The listing builds one solid part. Answer for the finished solid, in the listing's coordinates (mm). Face numbers are marked on the shaded views. A direction names the side the tool comes from. Give positions to 0.01 mm unless a question says otherwise; leave off trailing zeros. Write each loop counter-clockwise with the first axis right and the second up, starting at its lowest first coordinate (ties: lowest second). Pieces come first, ordered by that corner, then holes. Notation, with made-up numbers: (-23.75, 48.25) -> (-8.75, 48.25) arc R16 ccw to (-8.75, 53.25) -> close; hole circle Ø3 at (76.25, 68). An arc over 180 degrees is marked (long way). Use CSV: the item, a comma, the result in double quotes. Start each with the question number.
Autodesk Inventor part; units mm, degrees
ref_plane "Work Plane1" through (10, 0, 10) normal (0.7071, 0, -0.7071) x (0, -1, 0)
ref_plane "Work Plane2" through (0, -10, 0) normal (0, 1, 0) x (1, 0, 0)
ref_plane "YZ Plane" through (0, 0, 0) normal (1, 0, 0) x (0, 1, 0)
sketch "Sketch1" plane through (0, 0, 0) normal (0, 1, 0) x (-1, 0, 0)
  line L0 (10, -10) -> (-10, -10)
  line L1 (-10, -10) -> (-10, 10)
  line L2 (-10, 10) -> (10, 10)
  line L3 (10, 10) -> (10, -10)
  dimension "d0" = 20
  dimension "d1" = 20
extrude "Main Body Extrusion" add sketch "Sketch1" against normal blind 10
ref_plane "Work Plane1" through (10, 0, 10) normal (0.7071, 0, -0.7071) x (0, -1, 0)
sketch "Sketch2" plane through (10, 0, 10) normal (0.7071, 0, -0.7071) x (0, -1, 0)
  line L0 (0, 0) -> (10, 0)
  line L1 (10, 14.1421) -> (10, 28.2843)
  line L2 (5, 0) -> (10, 28.2843)
  line L3 (5, 0) -> (10, 0)
  line L4 (10, 0) -> (10, 14.1421)
  line L5 (10, 14.1421) -> (10, 0)
  point P0 (0, 14.1421)
extrude "Slanted Cut" cut sketch "Sketch2" along normal through all both and the other way through all
sketch "Sketch3" plane through (0, 0, 0) normal (0, 1, 0) x (1, 0, 0)
  point P0 (0, 0)
  point P1 (0, 0)
hole "Screw Hole" at (0, 0, 0) direction (0, -1, 0) diameter 4.2 end through all
ref_plane "Work Plane2" through (0, -10, 0) normal (0, 1, 0) x (1, 0, 0)
sketch "Sketch4" plane through (0, -10, 0) normal (0, 1, 0) x (1, 0, 0)
  circle A0 centre (0, 0) radius 4
  dimension "d14" = 8
extrude "Counterbore for Screw Hole" cut sketch "Sketch4" along normal blind 7.5
sketch "Sketch5" plane through (0, 0, 0) normal (0, 1, 0) x (1, 0, 0)
  line L0 (-10, -10) -> (10, -10)
  line L1 (3, -10) -> (-3, -10)
  line L2 (-3, -10) -> (-3, 10)
  line L3 (-3, 10) -> (3, 10)
  line L4 (3, 10) -> (3, -10)
  circle A0 centre (0, 0) radius 2.1
  line L5 (3, 10) -> (-3, 10)
  line L6 (-3, 10) -> (-3, 6)
  line L7 (-3, 6) -> (3, 6)
  line L8 (3, 6) -> (3, 10)
  line L9 (3, -10) -> (-3, -10)
  line L10 (-3, -10) -> (-3, -6)
  line L11 (-3, -6) -> (3, -6)
  line L12 (3, -6) -> (3, -10)
extrude "Alignment Extrusion" add sketch "Sketch5" along normal blind 3 contours L2 L11 L4 L0 | L2 L3 L4 L7
properties part number "corner_3DPrint"
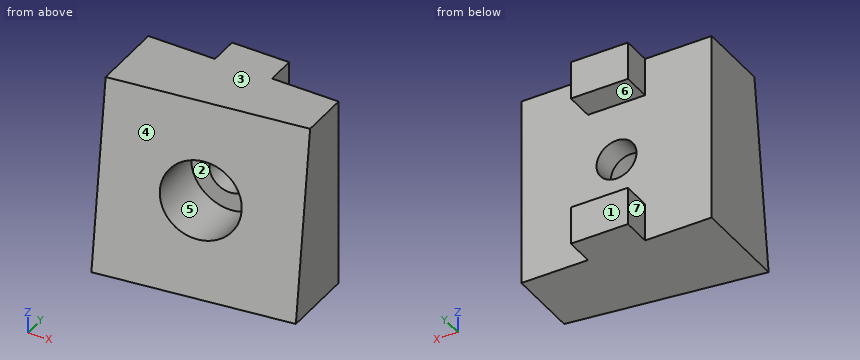
Q1. The mould has two halves that part along Z. Classify the marked faces 1, 2 and 3: +Z half, -Z half, draft (parallel to the pull), parting line (faces both ways), or undercut.
Q2. Section C-C on y = 0.75 is taken. Give the vertices of the cut face in (x, z), then the cut area to 3 significant figures.
Q3. Section B-B on z = 0 is taken. Give the vertices of the cut face in (x, y), then the cut area to 3 significant figures.
Q4. For the marked faces 4, 5, 6 and 7, determine the directions among +Z, -Z, +X, -X, +Y, -Y from which every point of the face is accessible in a straight line to the end or side of a thin tool.
Q5. Straight lines are drawn through the part: L1, parallel to X at y = -0.6, z = 0; L2, parallel to X at y = -4.8, z = 0. For each, find the intervals that lie inside material, in ascending order.
Q6. Section D-D on y = -1.75 is taken. Give the vertices of the cut face in (x, z).
Q7. Section A-A on x = 0 is taken. Give the vertices of the cut face in (y, z).
Q8. Flat-ended cylindrical pins translate along their axes: pin 1 Ø3 at (y, z) = (-8, 6.5) entering from -X; pin 2 Ø0.9 at (y, z) = (1, 7.5) entering from -X; pin 3 Ø2 at (x, z) = (1, -2.5) entering from +Y; pin 4 Ø2 at (x, z) = (-7, -0.5) entering from -Y. Find the tip coordinate at first contact, or state that the pin passes through.
Output:
1,face 1,"draft"
1,face 2,"undercut"
1,face 3,"+Z half"
2,outline,"(-3, -10) -> (3, -10) -> (3, -6) -> (-3, -6) -> close; (-3, 6) -> (3, 6) -> (3, 10) -> (-3, 10) -> close"
2,area,"48.0 mm²"
3,outline,"(-10, -8.75) -> (-4, -8) -> (-4, -2.5) -> (-2.1, -2.5) -> (-2.1, 0) -> (-10, 0) -> close; (2.1, -2.5) -> (4, -2.5) -> (4, -7) -> (10, -6.25) -> (10, 0) -> (2.1, 0) -> close"
3,area,"99.5 mm²"
4,face 4,"+Z, +X, -Y"
4,face 5,"-Y"
4,face 6,"+X, -X, +Y"
4,face 7,"+Z, -Z, -X, +Y"
5,L1,"-10 to -2.1, 2.1 to 10"
5,L2,"-10 to -4, 4 to 10"
6,outline,"(-10, -10) -> (10, -10) -> (10, 10) -> (-10, 10) -> close; hole circle Ø4.2 at (0, 0)"
7,outline,"(-8.75, -10) -> (3, -10) -> (3, -6) -> (0, -6) -> (0, -2.1) -> (-2.5, -2.1) -> (-2.5, -4) -> (-8, -4) -> close; (-7, 4) -> (-2.5, 4) -> (-2.5, 2.1) -> (0, 2.1) -> (0, 6) -> (3, 6) -> (3, 10) -> (-6.25, 10) -> close"
8,pin 1,"x = -10"
8,pin 2,"x = -3"
8,pin 3,"y = 0"
8,pin 4,"y = -8.61"
